Source: CAD feature listing. Evaluate the final solid. Frame: model axes, mm. A direction names the side the tool comes from. Coordinates: 2 decimals unless noted, no trailing zeros. Loops run counter-clockwise (first coordinate to the right, second up) from the corner with the lowest first, then second, coordinate; pieces in that order, holes last.
from build123d import *

# Parameters (mm, degrees)
F0_W     = 53.975
F0_H     = 46.0375
F1_DEPTH = 29.5275
F2_T     = -4.7625
F4_D     = 17.78
F4_DEPTH = 25.4


with BuildPart() as f1:
    # F0 (on Front) → F1 (new body)
    with BuildSketch(Plane.XZ):
        with Locations((26.9875, 23.01875)):
            Rectangle(F0_W, F0_H)
    extrude(amount=F1_DEPTH)

    # F2
    f2_openings = [f1.faces().sort_by_distance(p)[0] for p in [
        (26.9875, -29.5275, 23.01875),
    ]]
    offset(amount=F2_T, openings=f2_openings)

    # F4
    with Locations(Plane(origin=(0, 0, 0), x_dir=(-1, 0, 0), z_dir=(0, 1, 0))):
        with Locations((-26.9875, 23.01875)):
            Hole(F4_D / 2, depth=F4_DEPTH)


solid = f1.part
Q1. Section C-C, the plane z = 27.5. Return the cut outline in (x, y) (1 decimal), plus the area to 3 significant figures.
Q2. Section D-D, the plane x = 46. Return the cut outline in (y, z) (1 decimal).
Q3. Section A-A, the plane x = 27. Return the cut outline in (y, z) (1 decimal), plus the area to 3 significant figures.
Q4. Contact query for a flat-ended pin moving along its axis: pin 1 Ø11 at (x, z) = (16.5, 15) entering from -Y. Output: stop coordinate, or through.
Q5. Access query for faces 1 (the flat face through (49.212, -17, 23)), 2 (the flat face through (27, -29.528, 3)). Directions: +Z, -Z, +X, -X, +Y, -Y. A direction counts if a zero-diameter tool reaches every point of the face in a straight line with its end or side. Return the directions, or none.
Q6. Line query: line 1 along Z through (x, y) = (22, -17.5) (1 decimal); line 2 along X through (y, z) = (-28, 25.5) (1 decimal); line 3 along Y through (x, z) = (33, 8). Output: solid intervals per line, ascending.
Q7. Draft query along X for faces 3 (the flat face through (4.762, -17, 23)), 4 (the flat face through (53.975, -15, 23)), 5 (the flat face through (27, -15, 46.038)), 6 (the flat face through (0, -15, 23)). Return one class per face: +X half, -X half, draft (parallel to the pull), parting line (faces both ways), or undercut.
Q8. Section B-B, the plane y = -25. Return the cut outline in (x, z) (1 decimal).
Derived:
1. outline: (0, -29.5) - (4.8, -29.5) - (4.8, -4.8) - (19.3, -4.8) - (19.3, 0) - (0, 0) - close; (34.7, -4.8) - (49.2, -4.8) - (49.2, -29.5) - (54, -29.5) - (54, 0) - (34.7, 0) - close
1. area: 420 mm2
2. outline: (-29.5, 0) - (0, 0) - (0, 46) - (-29.5, 46) - (-29.5, 41.3) - (-4.8, 41.3) - (-4.8, 4.8) - (-29.5, 4.8) - close
3. outline: (-29.5, 0) - (0, 0) - (0, 14.1) - (-4.8, 14.1) - (-4.8, 4.8) - (-29.5, 4.8) - close; (-29.5, 41.3) - (-4.8, 41.3) - (-4.8, 31.9) - (0, 31.9) - (0, 46) - (-29.5, 46) - close
3. area: 370 mm2
4. pin 1: stops at y = -4.76
5. face 1: -Y
5. face 2: +Z, -Z, +X, -X, -Y
6. line 1: z = 0 to 4.8, 41.3 to 46
6. line 2: x = 0 to 4.8, 49.2 to 54
6. line 3: y = -4.76 to 0
7. face 3: undercut
7. face 4: +X half
7. face 5: draft
7. face 6: -X half
8. outline: (0, 0) - (54, 0) - (54, 46) - (0, 46) - close; hole (4.8, 4.8) - (49.2, 4.8) - (49.2, 41.3) - (4.8, 41.3) - close
